from build123d import *

# Parameters (mm, degrees)
F0_R     = 11
F0_W     = 50
F0_H     = 6
F1_DEPTH = 5
F2_DEPTH = 40


with BuildPart() as f1:
    # F0 (on Front) → F1 (new body, symmetric)
    with BuildSketch(Plane.XZ):
        with BuildLine():
            Line((-25, 44), (-25, 0))
            ThreePointArc((-25, 0), (0, -25), (25, 0))
            Line((25, 0), (25, 44))
            Line((25, 44), (-25, 44))
        make_face()
        Circle(F0_R, mode=Mode.SUBTRACT)
        with Locations((0, 47)):
            Rectangle(F0_W, F0_H)
    extrude(amount=F1_DEPTH, both=True)

    # F0 (on Front) → F2 (join, symmetric)
    with BuildSketch(Plane.XZ):
        with Locations((0, 47)):
            Rectangle(F0_W, F0_H)
    extrude(amount=F2_DEPTH, both=True)


solid = f1.part
Work out the finished part from the listing and answer in its coordinate system (mm). A direction names the side the tool comes from. Give positions to 0.01 mm unless a question says otherwise; leave off trailing zeros. Write each loop counter-clockwise with the first axis right and the second up, starting at its lowest first coordinate (ties: lowest second). Pieces come first, ordered by that corner, then holes. Notation, with made-up numbers: (47.25, 72.5) - (71.25, 72.5) arc R30 ccw to (71.25, 108.5) - close; hole circle Ø1 at (-29, 2.25). An arc over 180 degrees is marked (long way). One line per item, written item: value. Start each with the question number.
1. Find section C-C (x = 20). Write down the section's boundary in (y, z), then the cut area to 3 significant figures.
2. Find section A-A (x = 0). Write down the section's boundary in (y, z), then the cut area to 3 significant figures.
3. Find section B-B (y = -1). Write down the section's boundary in (x, z), then the cut area to 3 significant figures.
4. Given pin 1 (5 mm diameter, centred on x = 11.5, z = 26.5, fed in from -Y); pin 2 (10 mm diameter, centred on x = 12.5, y = -13, fed in from -Z); pin 3 (4 mm diameter, centred on x = -2, y = 0, fed in from -Z), each flat-ended and moving along its own axis, determine where each tip first touches the part or whether it passes through.
5. Consider probe 1 along Z at (x, y) = (0, -1); probe 2 along Y at (x, z) = (15.5, -1); probe 3 along Z at (x, y) = (8.5, -17.5). Determine where each line is inside the solid, lowest interval first.
6. For a pull along Z with two mould halves and no side action, classify faces 1 (the cylindrical face through (-2.38, 0.07, -10.74)), 2 (the flat face through (0, -1, 50)), 3 (the flat face through (25, 0, 36)) as +Z half, -Z half, draft (parallel to the pull), parting line (faces both ways), or undercut.
7. For faces 4 (the flat face through (0, 5, 18)), 5 (the flat face through (0, -5, 18)), 6 (the flat face through (0, 40, 47)), determine the directions among +Z, -Z, +X, -X, +Y, -Y from which every point of the face is accessible in a straight line to the end or side of a thin tool.
8. Find section D-D (z = 34). Write down the section's boundary in (x, y), then the cut area to 3 significant figures.
Geometry results:
1. outline: (-40, 44) - (-5, 44) - (-5, -15) - (5, -15) - (5, 44) - (40, 44) - (40, 50) - (-40, 50) - close
1. area: 1,070 mm2
2. outline: (-40, 44) - (-5, 44) - (-5, 11) - (5, 11) - (5, 44) - (40, 44) - (40, 50) - (-40, 50) - close; (-5, -25) - (5, -25) - (5, -11) - (-5, -11) - close
2. area: 950 mm2
3. outline: (-25, 0) arc R25 ccw to (25, 0) - (25, 50) - (-25, 50) - close; hole circle Ø22 at (0, 0)
3. area: 3,100 mm2
4. pin 1: y = -5
4. pin 2: z = 44
4. pin 3: z = -25
5. probe 1: -25 to -11, 11 to 50
5. probe 2: -5 to 5
5. probe 3: 44 to 50
6. face 1: undercut
6. face 2: +Z half
6. face 3: draft
7. face 4: -Z, +X, -X, +Y
7. face 5: -Z, +X, -X, -Y
7. face 6: +Z, -Z, +X, -X, +Y
8. outline: (-25, -5) - (25, -5) - (25, 5) - (-25, 5) - close
8. area: 500 mm2
